Can you work these out from the model? Positions are in its coordinate system, mm. Face numbers are marked on the shaded views. Round coordinates to 2 decimals unless told otherwise and drop trailing zeros. Order: outer loops, then holes, each group sorted by start corner. A loop starts at its lowest first (then second) coordinate and runs counter-clockwise, first axis right, second up. Notation, with made-up numbers: (48, 23.25) - (65, 23.25) arc R10 cw to (65, 31.25) - close; hole circle Ø5 at (14, 15.5). An arc over 180 degrees is marked (long way). Write item = value, one per line.
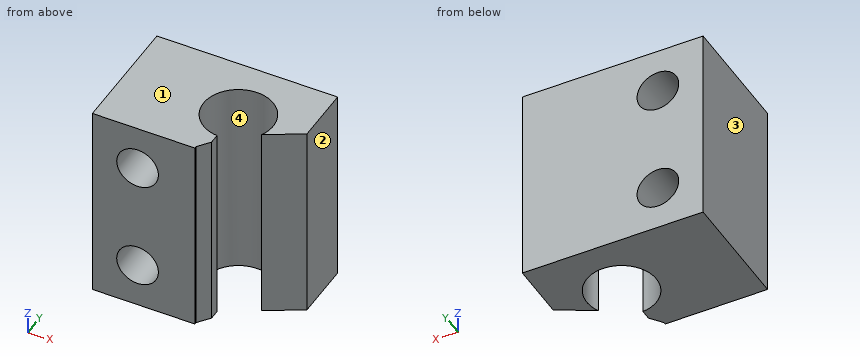
from build123d import *

# Parameters (mm, degrees)
F1_DEPTH = 29
F2_R     = 3
F3_DEPTH = 17.501


with BuildPart() as f1:
    # F0 (on Top) → F1 (new body)
    with BuildSketch(Plane.XY):
        with BuildLine():
            ThreePointArc((1.397452, -3.25215), (-0.64173, 6.074606), (6.33527, -0.44215))
            Line((6.33527, -0.44215), (11.331258, 2.423141))
            Line((11.331258, 2.423141), (11.331258, 10.728996))
            Line((11.331258, 10.728996), (-14.668742, 10.728996))
            Line((-14.668742, 10.728996), (-14.668742, -6.771004))
            Line((-14.668742, -6.771004), (0.066813, -6.771004))
            Line((0.066813, -6.771004), (0.066813, -6.465031))
            Line((0.066813, -6.465031), (1.397452, -4.728965))
            Line((1.397452, -4.728965), (1.397452, -3.25215))
        make_face()
    extrude(amount=F1_DEPTH)

    # F2 (on face) → F3 (cut, through all)
    with BuildSketch(Plane(origin=(0, 10.728996, 0), x_dir=(-1, 0, 0), z_dir=(0, 1, 0))):
        with Locations((8.168742, 22.5)):
            Circle(F2_R)
        with Locations((8.168742, 6.5)):
            Circle(F2_R)
    extrude(amount=-F3_DEPTH, mode=Mode.SUBTRACT)


solid = f1.part
(1) If we section it at A-A (z = 6.5): Write out the boundary of the cut face in (x, y).
Computed:
outline = (-14.67, -6.77) - (-11.17, -6.77) - (-11.17, 10.73) - (-14.67, 10.73) - close; (-5.17, -6.77) - (0.07, -6.77) - (0.07, -6.47) - (1.4, -4.73) - (1.4, -3.25) arc R5 cw (long way) to (6.34, -0.44) - (11.33, 2.42) - (11.33, 10.73) - (-5.17, 10.73) - close
(2) If we section it at C-C (x = -0.5): Write out the boundary of the cut face in (y, z).
Computed:
outline = (-6.77, 0) - (-2.69, 0) - (-2.69, 29) - (-6.77, 29) - close; (6.15, 0) - (10.73, 0) - (10.73, 29) - (6.15, 29) - close
(3) Thinking about a two-plate mould opening in X: for the marked faces 1, 2, 3 and 4, which applies, +X half, -X half, draft (parallel to the pull), parting line (faces both ways), or undercut?
Computed:
face_1 = draft
face_2 = +X half
face_3 = -X half
face_4 = undercut
(4) If we section it at B-B (y = 4): Write out the boundary of the cut face in (x, z), plus the area to 3 significant figures.
Computed:
outline = (-14.67, 0) - (-2.62, 0) - (-2.62, 29) - (-14.67, 29) - close; (6.29, 0) - (11.33, 0) - (11.33, 29) - (6.29, 29) - close; hole circle Ø6 at (-8.17, 6.5); hole circle Ø6 at (-8.17, 22.5)
area = 439 mm^2
(5) If we section it at D-D (y = -2.25): Write out the boundary of the cut face in (x, z), plus the area to 3 significant figures.
Computed:
outline = (-14.67, 0) - (-1.2, 0) - (-1.2, 29) - (-14.67, 29) - close; hole circle Ø6 at (-8.17, 6.5); hole circle Ø6 at (-8.17, 22.5)
area = 334 mm^2
(6) If I drill on line 1 (Z direction, x = -5.5, y = 9.25); line 2 (Z direction, x = -10, y = 1.5); line 3 (Y direction, x = 1.75, z = 20.25), over which ranges is the centre line in solid material (lowest first)? Write a range as from..to.
Computed:
line_1 = 0..5.13, 7.87..21.13, 23.87..29
line_2 = 0..4.12, 8.88..20.12, 24.88..29
line_3 = 6.73..10.73
(7) Will these pins go through, and if not, where does the flat tip stop? P1, Ø10, axis at x = 4, y = -3.5, coming from the +Z side; P2, Ø0.7, axis at y = -4, z = 10, coming from the +X side.
Computed:
P1 = 29
P2 = 1.4
